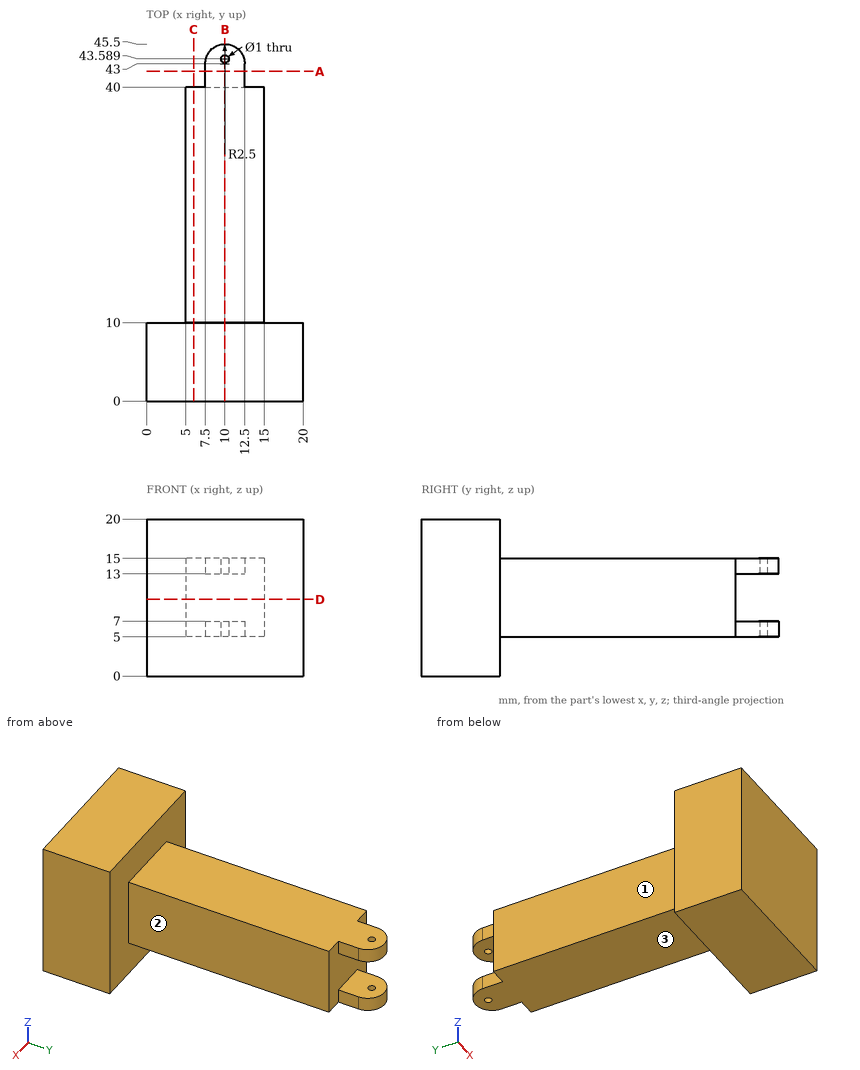
For this review, use the dimensioned drawing (mm, ordinates from the lowest corner) and the shaded views. A direction names the side the tool comes from. Give positions to 0.01 mm unless a question says otherwise; leave off trailing zeros. Order: outer loops, then holes, each group sorted by start corner. A loop starts at its lowest first (then second) coordinate and runs counter-clockwise, first axis right, second up. Notation, with made-up numbers: (85, -8.5) - (93, -8.5) arc R8 ccw to (93, 2.5) - close; hole circle Ø3 at (41, 86.25). An arc over 180 degrees is marked (long way). Use CSV: the item, a comma, the result in double quotes. Start each with the question number.
Q1. For line 1 (Z direction, x = 9.5, y = 42.5); line 2 (X direction, y = 23, z = 10.75); line 3 (Y direction, x = 16, z = 11.25), list the stretches that pass through material, from the lowest coordinate up.
Q2. For P1, Ø4, axis at x = 3.5, y = 35, coming from the +Z side; P2, Ø12, axis at x = 17, y = 6, coming from the -Z side; P3, Ø2, axis at y = 42, z = 13.5, coming from the -X side; P4, Ø1.5, axis at y = 15.5, z = 11, coming from the -X side, all flat-tipped, find the tip position at first contact; note any pin that passes through.
Q3. Take a section at A-A (y = 42). State the section outline as (x, z) points, and give its area (3 significant figures).
Q4. Take a section at C-C (x = 6). State the section outline as (y, z) points, and give its area (3 significant figures).
Q5. Take a section at D-D (z = 9.75). State the section outline as (x, y) points, and give its area (3 significant figures).
Q6. Take a section at B-B (x = 10). State the section outline as (y, z) points.
Q7. Machinability: for the marked faces 1, 2 and 3, which of the approach directions +Z, -Z, +X, -X, +Y, -Y give a long, thin tool a straight path to every point of the face, cutting with its end or side? Answer none if there is none.
Calculated:
1,line 1,"z = 5 to 7, 13 to 15"
1,line 2,"x = 5 to 15"
1,line 3,"y = 0 to 10"
2,P1,"stops at z = 15"
2,P2,"stops at z = 0"
2,P3,"stops at x = 7.5"
2,P4,"stops at x = 5"
3,outline,"(7.5, 5) - (12.5, 5) - (12.5, 7) - (7.5, 7) - close; (7.5, 13) - (12.5, 13) - (12.5, 15) - (7.5, 15) - close"
3,area,"20.0 mm²"
4,outline,"(0, 0) - (10, 0) - (10, 5) - (40, 5) - (40, 15) - (10, 15) - (10, 20) - (0, 20) - close"
4,area,"500 mm²"
5,outline,"(0, 0) - (20, 0) - (20, 10) - (15, 10) - (15, 40) - (5, 40) - (5, 10) - (0, 10) - close"
5,area,"500 mm²"
6,outline,"(0, 0) - (10, 0) - (10, 5) - (43.09, 5) - (43.09, 7) - (40, 7) - (40, 13) - (43.09, 13) - (43.09, 15) - (10, 15) - (10, 20) - (0, 20) - close; (44.09, 5) - (45.5, 5) - (45.5, 7) - (44.09, 7) - close; (44.09, 13) - (45.5, 13) - (45.5, 15) - (44.09, 15) - close"
7,face 1,"+Z, -Z, -X, +Y"
7,face 2,"+Z, -Z, +X, +Y"
7,face 3,"-Z, +X, -X, +Y"
